Can you work these out from the model? Positions are in its coordinate system, mm. A direction names the side the tool comes from. Give positions to 0.01 mm unless a question says otherwise; leave off trailing zeros. Order: outer loops, then holes, each group sorted by start corner. A loop starts at its lowest first (then second) coordinate and runs counter-clockwise, first axis right, second up. Notation, with made-up numbers: M 58.25,-16 L 74.25,-16 A33 cw 74.25,15 Z; hole C -2,60.25 d5. An arc over 180 degrees is marked long. Use a Markdown table: item, result. Add a question column.
from build123d import *

# Parameters (mm, degrees)
SKETCH2_R           = 12.7
BOSS_EXTRUDE1_DEPTH = 101.6
BOSS_EXTRUDE2_DEPTH = 12.7
SKETCH4_R           = 14.196290171
CUT_EXTRUDE1_DEPTH  = 25.4


with BuildPart() as part:
    # Sketch2 → Boss-Extrude1 (new body)
    with BuildSketch(Plane.XY):
        Circle(SKETCH2_R)
    extrude(amount=BOSS_EXTRUDE1_DEPTH)

    # Sketch3 → Boss-Extrude2 (add)
    with BuildSketch(Plane.XY.offset(101.6)):
        with BuildLine():
            ThreePointArc((-8.89, 0), (-6.35, -2.54), (-3.81, 0))
            Line((-3.81, 0), (-8.89, 0))
        make_face()
        with BuildLine():
            Line((-8.89, 0), (-3.81, 0))
            ThreePointArc((-3.81, 0), (-6.35, 2.54), (-8.89, 0))
        make_face()
        with BuildLine():
            ThreePointArc((8.89, 0), (6.35, 2.54), (3.81, 0))
            Line((3.81, 0), (8.89, 0))
        make_face()
        with BuildLine():
            Line((8.89, 0), (3.81, 0))
            ThreePointArc((3.81, 0), (6.35, -2.54), (8.89, 0))
        make_face()
    extrude(amount=BOSS_EXTRUDE2_DEPTH)

    # Sketch4 → Cut-Extrude1 (cut)
    with BuildSketch(Plane(origin=(0, 0, 0), x_dir=(-1, 0, 0), z_dir=(0, 0, -1))):
        Circle(SKETCH4_R)
    extrude(amount=-CUT_EXTRUDE1_DEPTH, mode=Mode.SUBTRACT)


solid = part.part
1. If we section it at C-C, the plane x = 7: List the corners of the cut face in (y, z) for me, then the cut area to 3 significant figures.
2. If we section it at A-A, the plane y = 0: List the corners of the cut face in (x, z) for me, then the cut area to 3 significant figures.
3. If we section it at B-B, the plane z = 73.5: List the corners of the cut face in (x, y) for me, then the cut area to 3 significant figures.
4. We'd pull the mould along X, two halves only. Please class faces 3 (the face through (-2.75, -12.4, 62.97)), 4 (the face through (8.22, -1.72, 107.86)), 5 (the face through (0, 0, 25.4)): +X half, -X half, draft (parallel to the pull), parting line (faces both ways), or undercut.
5. If we section it at D-D, the plane x = 0: List the corners of the cut face in (y, z) for me.
6. On a 3-axis mill with a long thin cutter (end or side, diameter ignored), from which of +Z, -Z, +X, -X, +Y, -Y can I reach the whole of each face in a straight line? I mean faces 1 (the face through (6, 0, 114.3)), 2 (the face through (-8.22, 1.72, 107.86)). Say none if no direction works.
7. I need wall thicknesses on L1, parallel to Z at x = 6.75, y = 3; L2, parallel to Y at x = 0, z = 48; L3, parallel to X at y = 8.5, z = 63. Which ranges of each line are inside material? Lowest first, please. Write a range as [from, to].
8. Will these pins go through, and if not, where does the flat tip stop? pin 1 (6 mm diameter, centred on x = -6, z = 55, fed in from -Y); pin 2 (1.5 mm diameter, centred on x = -6, z = 69.5, fed in from -Y); pin 3 (8 mm diameter, centred on x = -7, z = 100.5, fed in from +Y).
Geometry results:
| question | item | result |
|---|---|---|
| 1 | outline | M -10.6,25.4 L 10.6,25.4 L 10.6,101.6 L 2.46,101.6 L 2.46,114.3 L -2.46,114.3 L -2.46,101.6 L -10.6,101.6 Z |
| 1 | area | 1,680 mm^2 |
| 2 | outline | M -12.7,25.4 L 12.7,25.4 L 12.7,101.6 L 8.89,101.6 L 8.89,114.3 L 3.81,114.3 L 3.81,101.6 L -3.81,101.6 L -3.81,114.3 L -8.89,114.3 L -8.89,101.6 L -12.7,101.6 Z |
| 2 | area | 2,060 mm^2 |
| 3 | outline | C 0,0 d25.4 |
| 3 | area | 507 mm^2 |
| 4 | face 3 | parting line |
| 4 | face 4 | undercut |
| 4 | face 5 | draft |
| 5 | outline | M -12.7,25.4 L 12.7,25.4 L 12.7,101.6 L -12.7,101.6 Z |
| 6 | face 1 | +Z, +X, -X, +Y, -Y |
| 6 | face 2 | +Z |
| 7 | L1 | z = [25.4, 101.6] |
| 7 | L2 | y = [-12.7, 12.7] |
| 7 | L3 | x = [-9.44, 9.44] |
| 8 | pin 1 | stops at y = -12.34 |
| 8 | pin 2 | stops at y = -11.56 |
| 8 | pin 3 | stops at y = 12.34 |
